Check sheet for the drawn part. Datum: minimum x, y, z corner. Units: mm. Give positions to 0.01 mm unless a question says otherwise; leave off trailing zeros. Order: outer loops, then holes, each group sorted by start corner. A loop starts at its lowest first (then second) coordinate and runs counter-clockwise, first axis right, second up. Notation, with made-up numbers: (-18.75, 27) -> (-6.75, 27) arc R12 cw to (-6.75, 38) -> close; hole circle Ø7 at (-24, 58). An arc over 180 degrees is marked (long way). Return JSON: item names as keys, results as strings. Group by question number.
(1) Release check for a two-part mould opening along Y. For the marked faces 1 and 2 record: pulls with the +Y half, pulls with the -Y half, needs draft (parallel to the pull), parting line crosses it, or undercut.
(2) Cross-section at C-C on x = 10.5. Enter the section's corners in (y, z), then the cut area to 3 significant figures.
(3) Thickness scan on line 1 along Y through (x, z) = (14, 210); line 2 along Z through (x, y) = (3, 181.5); line 3 along Y through (x, z) = (10, 269). Record the ranges inside material, lowest first.
(4) Depth check by flat-ended pin: pin 1 Ø5 at (x, z) = (5.5, 303) entering from +Y; pin 2 Ø12 at (x, z) = (12, 447) entering from +Y; pin 3 Ø10 at (x, y) = (14.5, 67.5) entering from -Z. Enter the tip coordinate at first touch or a pass-through.
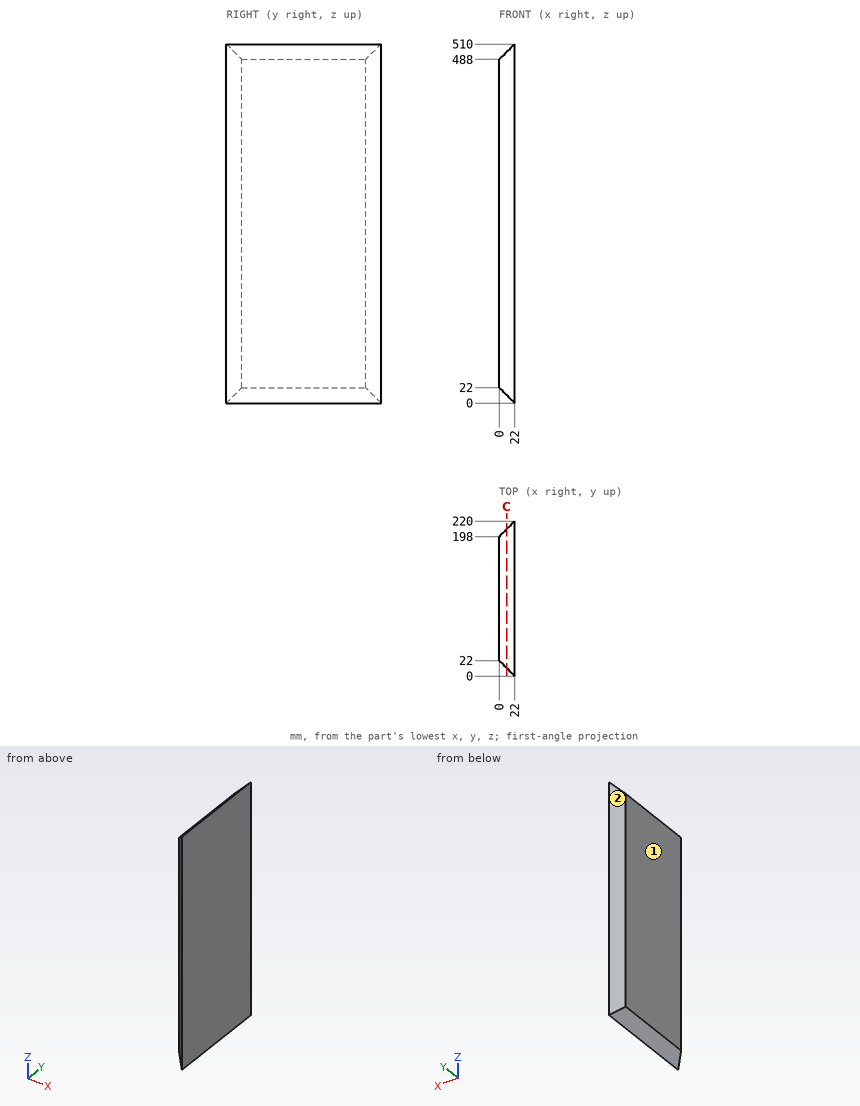
Verdict:
{
 "1": {"face 1": "needs draft", "face 2": "pulls with the +Y half"},
 "2": {"outline": "(11.5, 11.5) -> (208.5, 11.5) -> (208.5, 498.5) -> (11.5, 498.5) -> close", "area": "95,900 mm²"},
 "3": {"line 1": "8 to 212", "line 2": "19 to 491", "line 3": "12 to 208"},
 "4": {"pin 1": "y = 206", "pin 2": "y = 216", "pin 3": "z = 2.5"}
}
